```python
from build123d import *

# Parameters (mm, degrees)
SKETCH1_R           = 1.075
BOSS_EXTRUDE1_DEPTH = 3.9
CUT_EXTRUDE1_DEPTH  = 1
CUT_EXTRUDE2_START  = -1
SKETCH4_R           = 2.75
SKETCH4_R_2         = 1.075
CUT_EXTRUDE2_DEPTH  = 1
SKETCH6_W           = 10
SKETCH6_H           = 3.9
BOSS_EXTRUDE2_DEPTH = 5
SKETCH7_W           = 10
SKETCH7_H           = 3.9
BOSS_EXTRUDE3_DEPTH = 10
SKETCH10_R          = 1.5
CUT_EXTRUDE3_DEPTH  = 10
FILLET2_R           = 3
FILLET3_R           = 1
FILLET4_R           = 2
FILLET5_R           = 4
CHAMFER1_SIZE       = 0.6
FILLET6_R           = 0.5
FILLET7_R           = 0.2


with BuildPart() as part:
    # Sketch1 → Boss-Extrude1 (new body)
    with BuildSketch(Plane(origin=(0, 0, 0), x_dir=(1, 0, 0), z_dir=(0, 1, 0))):
        Polygon((-4.075, 0), (-4.075, 7.5), (7.425, 15.5), (7.425, -15.5), (-4.075, -7.5), align=None)
        with Locations(Location((0, 0, 0), (0, 0, 270))):
            Circle(SKETCH1_R, mode=Mode.SUBTRACT)
    extrude(amount=BOSS_EXTRUDE1_DEPTH)

    # Sketch2 → Cut-Extrude1 (cut)
    with BuildSketch(Plane.XZ):
        with BuildLine():
            ThreePointArc((-4.075, 0), (-2.683757211, 3.358757211), (0.675, 4.75))
            Line((0.675, 4.75), (-4.075, 4.75))
            Line((-4.075, 4.75), (-4.075, 0))
        make_face()
        with BuildLine():
            Line((-4.075, -4.75), (0.675, -4.75))
            ThreePointArc((0.675, -4.75), (-2.683757211, -3.358757211), (-4.075, 0))
            Line((-4.075, 0), (-4.075, -4.75))
        make_face()
        with BuildLine():
            ThreePointArc((-1.075, 0), (0, 1.075), (1.075, 0))
            Line((1.075, 0), (5.425, 0))
            ThreePointArc((5.425, 0), (4.033757211, 3.358757211), (0.675, 4.75))
            ThreePointArc((0.675, 4.75), (-2.683757211, 3.358757211), (-4.075, 0))
            Line((-4.075, 0), (-1.075, 0))
        make_face()
        with BuildLine():
            Line((5.425, 0), (1.075, 0))
            ThreePointArc((1.075, 0), (0, -1.075), (-1.075, 0))
            Line((-1.075, 0), (-4.075, 0))
            ThreePointArc((-4.075, 0), (-2.683757211, -3.358757211), (0.675, -4.75))
            ThreePointArc((0.675, -4.75), (4.033757211, -3.358757211), (5.425, 0))
        make_face()
    extrude(amount=-CUT_EXTRUDE1_DEPTH, mode=Mode.SUBTRACT)

    # Sketch4 → Cut-Extrude2 (cut)
    # profile 1 of 2: a face of its own
    with BuildSketch(Plane(origin=(0, 3.9, 0), x_dir=(1, 0, 0), z_dir=(0, 1, 0)).offset(CUT_EXTRUDE2_START)):
        with BuildLine():
            ThreePointArc((0, -2.75), (-2.75, 0), (0, 2.75))
            Line((0, 2.75), (-4.075, 2.75))
            Line((-4.075, 2.75), (-4.075, -2.75))
            Line((-4.075, -2.75), (0, -2.75))
        make_face()
    # profile 2 of 2: a face of its own
    with BuildSketch(Plane(origin=(0, 3.9, 0), x_dir=(1, 0, 0), z_dir=(0, 1, 0)).offset(CUT_EXTRUDE2_START)):
        Circle(SKETCH4_R)
        with Locations(Location((0, 0, 0), (0, 0, 90))):
            Circle(SKETCH4_R_2, mode=Mode.SUBTRACT)
    extrude(amount=CUT_EXTRUDE2_DEPTH, mode=Mode.SUBTRACT)

    # Sketch6 → Boss-Extrude2 (add)
    with BuildSketch(Plane(origin=(7.425, 0, 0), x_dir=(0, 0, -1), z_dir=(1, 0, 0))):
        with Locations((-2.5, 1.95)):
            Rectangle(SKETCH6_W, SKETCH6_H)
    extrude(amount=BOSS_EXTRUDE2_DEPTH)

    # Sweep1: sweep along a path in Sketch8
    with BuildLine(Plane.XY) as sweep1_path:
        Line((12.425, 1.95), (13.960898385, 1.95))
        ThreePointArc((13.960898385, 1.95), (15.692949192, 0.95), (15.692949192, -1.05))
        Line((15.692949192, -1.05), (10.525664283, -10))
    # Sketch7 → Sweep1 (sweep)
    with BuildSketch(Plane(origin=(12.425, 0, 0), x_dir=(0, 0, -1), z_dir=(1, 0, 0))):
        with Locations((-2.5, 1.95)):
            Rectangle(SKETCH7_W, SKETCH7_H)
    sweep(path=sweep1_path.line)

    # Sketch9 → Boss-Extrude3 (add)
    with BuildSketch(Plane(origin=(0, 0, -2.5), x_dir=(-1, 0, 0), z_dir=(0, 0, -1))):
        Polygon((-12.214413821, -10.975), (8.089101615, -10.975), (8.089101615, -9.025), (-24.910898385, -9.025), (-24.910898385, -10.975), align=None)
    extrude(amount=-BOSS_EXTRUDE3_DEPTH)

    # Sketch10 → Cut-Extrude3 (cut)
    with BuildSketch(Plane.XZ.offset(10.975)):
        with Locations(Location((-4.089101615, 2.5, 0), (0, 0, 270))):
            Circle(SKETCH10_R)
        with Locations(Location((20.910898385, 2.5, 0), (0, 0, 270))):
            Circle(SKETCH10_R)
    extrude(amount=-CUT_EXTRUDE3_DEPTH, mode=Mode.SUBTRACT)

    # Fillet2
    fillet2_edges = [part.edges().sort_by_distance(p)[0] for p in [
        (-4.075, 1.95, -7.5),
        (-4.075, 1.95, 7.5),
    ]]
    fillet(fillet2_edges, radius=FILLET2_R)

    # Fillet3
    fillet3_edges = [part.edges().sort_by_distance(p)[0] for p in [
        (-8.089101615, -10, -2.5),
        (24.910898385, -10, 7.5),
        (-8.089101615, -10, 7.5),
        (24.910898385, -10, -2.5),
    ]]
    fillet(fillet3_edges, radius=FILLET3_R)

    # Fillet4
    fillet4_edges = [part.edges().sort_by_distance(p)[0] for p in [
        (13.340246845, -9.025, 2.5),
    ]]
    fillet(fillet4_edges, radius=FILLET4_R)

    # Fillet5
    fillet5_edges = [part.edges().sort_by_distance(p)[0] for p in [
        (8.836914746, -9.025, 2.5),
    ]]
    fillet(fillet5_edges, radius=FILLET5_R)

    # Chamfer1
    chamfer1_edges = [part.edges().sort_by_distance(p)[0] for p in [
        (-4.089101615, -9.025, 4),
        (20.910898385, -9.025, 4),
    ]]
    chamfer(chamfer1_edges, length=CHAMFER1_SIZE)

    # Fillet6
    fillet6_edges = [part.edges().sort_by_distance(p)[0] for p in [
        (7.425, 1.95, -15.5),
        (7.425, 1.95, 15.5),
    ]]
    fillet(fillet6_edges, radius=FILLET6_R)

    # Fillet7
    fillet7_edges = [part.edges().sort_by_distance(p)[0] for p in [
        (24.910898385, -9.025, 2.5),
        (-0.280793973, -9.025, 7.5),
        (24.618005166, -9.025, -2.207106781),
        (24.618005166, -9.025, 7.207106781),
        (-0.280793973, -9.025, -2.5),
        (-8.089101615, -9.025, 2.5),
        (-7.796208396, -9.025, 7.207106781),
        (-7.796208396, -9.025, -2.207106781),
        (20.357623423, -9.025, 7.5),
        (20.357623423, -9.025, -2.5),
        (15.072297653, -8.025, 7.5),
        (15.072297653, -8.025, -2.5),
        (8.527513669, -8.489101615, -2.5),
        (8.527513669, -8.489101615, 7.5),
        (10.692949192, 3.9, 7.5),
        (10.692949192, 0, 7.5),
        (10.692949192, 0, -2.5),
        (10.692949192, 3.9, -2.5),
        (17.38169873, 1.925, 7.5),
        (14.004199655, -0.025, 7.5),
        (14.004199655, -0.025, -2.5),
        (17.38169873, 1.925, -2.5),
        (16.226998191, -4.025, 7.5),
        (11.99790747, -3.55, 7.5),
        (11.99790747, -3.55, -2.5),
        (16.226998191, -4.025, -2.5),
    ]]
    fillet(fillet7_edges, radius=FILLET7_R)


solid = part.part
```
Here's how the part is built. I have some questions about the finished solid (model axes, mm). A direction names the side the tool comes from. Coordinates: 2 decimals unless noted, no trailing zeros. Write each loop counter-clockwise with the first axis right and the second up, starting at its lowest first coordinate (ties: lowest second). Pieces come first, ordered by that corner, then holes. Notation, with made-up numbers: (24, 35) -> (76, 35) arc R7 ccw to (76, 41) -> close; hole circle Ø3 at (-13, 39.5). An arc over 180 degrees is marked (long way). Use a Markdown table: item, result. Add a question column.
(1) I'm going to push flat-ended pins straight in: P1, Ø4.5, axis at x = 12.5, y = -7, coming from the -Z side; P2, Ø1.6, axis at x = -1, z = 1, coming from the +Y side; P3, Ø1.1, axis at x = -2.5, y = 0.5, coming from the +Z side; P4, Ø2, axis at x = 11, z = -5, coming from the +Y side. Where does each tip first touch, or does it pass through?
(2) For faces 4 (the flat face through (19, -9.025, 1)), 5 (the flat face through (-4.075, 2, 0)), 6 (the flat face through (12, -6, -2.5)), 7 (the cylindrical face through (12.078, -3.531, 7.443)), which set-ups out of +Z, -Z, +X, -X, +Y, -Y let a thin tool reach every point of the face, with its end or its side?
(3) We'd pull the mould along Y, two halves only. Please class faces 1 (the flat face through (-1, -9.025, 2)), 2 (the cylindrical face through (-3.64, -10.31, 1.07)), 3 (the flat face through (9, -10.975, 2)): +Y half, -Y half, draft (parallel to the pull), parting line (faces both ways), or undercut.
(4) If we section it at A-A, the plane z = -13: Write out the boundary of the cut face in (x, y) (3 decimals).
(5) Please list where these lines run through material, in increasing order: line 1 (X direction, y = -10.5, z = 2.5); line 2 (Y direction, x = 1.5, z = 9); line 3 (Z direction, x = 10.5, y = -6.75).
(6) If we section it at B-B, the plane z = 10.5: Write out the boundary of the cut face in (x, y) (1 decimal).
Outcome:
| question | item | result |
|---|---|---|
| 1 | P1 | stops at z = -2.5 |
| 1 | P2 | stops at y = 2.9 |
| 1 | P3 | stops at z = 8.98 |
| 1 | P4 | passes through |
| 2 | face 4 | +Z, -Z, +X |
| 2 | face 5 | +Z, -Z, -X, +Y |
| 2 | face 6 | -Z, +X, -Y |
| 2 | face 7 | +Z, -X |
| 3 | face 1 | undercut |
| 3 | face 2 | draft |
| 3 | face 3 | -Y half |
| 4 | outline | (3.831, 0) -> (7.425, 0) -> (7.425, 3.9) -> (3.831, 3.9) -> close |
| 5 | line 1 | x = -8.09 to -5.59, -2.59 to 19.41, 22.41 to 24.91 |
| 5 | line 2 | y = 0 to 3.9 |
| 5 | line 3 | z = -2.5 to 7.5 |
| 6 | outline | (0.2, 0) -> (7.4, 0) -> (7.4, 3.9) -> (0.2, 3.9) -> close |
